Read the model definition and answer for the solid it produces. Units are mm, in the model's axes. Face numbers are marked on the shaded views. A direction names the side the tool comes from. Coordinates: 2 decimals unless noted, no trailing zeros. Order: outer loops, then holes, each group sorted by start corner. A loop starts at its lowest first (then second) coordinate and runs counter-clockwise, first axis right, second up.
```python
from build123d import *

# Parameters (mm, degrees)
SKETCH1_W           = 70.2
SKETCH1_H           = 17
SKETCH1_R           = 1.3
BOSS_EXTRUDE1_DEPTH = 1.6
SKETCH2_W           = 18.7
SKETCH2_H           = 15.5
SKETCH2_W_2         = 10.2
SKETCH2_H_2         = 14
BOSS_EXTRUDE2_DEPTH = 7.5
SKETCH3_W           = 52.2
SKETCH3_H           = 14.607054818
BOSS_EXTRUDE3_DEPTH = 2.4


with BuildPart() as part:
    # Sketch1 → Boss-Extrude1 (new body)
    with BuildSketch(Plane(origin=(0, 0, 0), x_dir=(1, 0, 0), z_dir=(0, 1, 0))):
        Rectangle(SKETCH1_W, SKETCH1_H)
        with Locations((-33.2, 6.6)):
            Circle(SKETCH1_R, mode=Mode.SUBTRACT)
        with Locations((33.2, 6.6)):
            Circle(SKETCH1_R, mode=Mode.SUBTRACT)
        with Locations((33.2, -6.6)):
            Circle(SKETCH1_R, mode=Mode.SUBTRACT)
        with Locations((-33.2, -6.6)):
            Circle(SKETCH1_R, mode=Mode.SUBTRACT)
    extrude(amount=-BOSS_EXTRUDE1_DEPTH)

    # Sketch2 → Boss-Extrude2 (add, symmetric)
    with BuildSketch(Plane.XY):
        with Locations((9.2, 7.75)):
            Rectangle(SKETCH2_W, SKETCH2_H)
        with Locations((25, 7)):
            Rectangle(SKETCH2_W_2, SKETCH2_H_2)
        with Locations((-25, 7)):
            Rectangle(SKETCH2_W_2, SKETCH2_H_2)
    extrude(amount=BOSS_EXTRUDE2_DEPTH, both=True)

    # Sketch3 → Boss-Extrude3 (add)
    with BuildSketch(Plane.XZ.offset(1.6)):
        Rectangle(SKETCH3_W, SKETCH3_H)
    extrude(amount=BOSS_EXTRUDE3_DEPTH)


solid = part.part
```
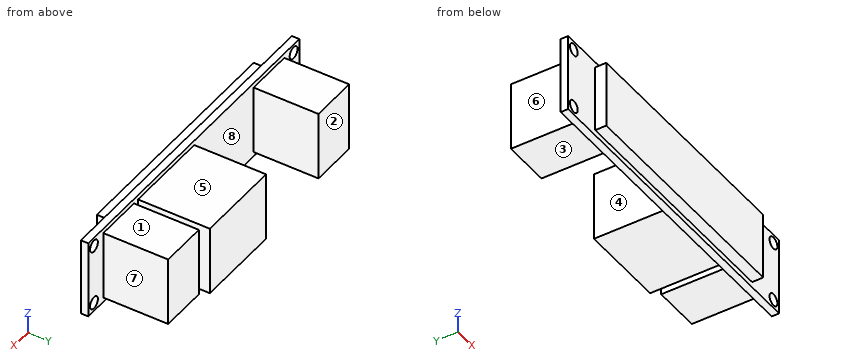
1) Flat-ended cylindrical pins translate along their axes: pin 1 Ø1.9 at (y, z) = (-2.5, 2) entering from -X; pin 2 Ø1.9 at (y, z) = (-3, -1.5) entering from +X; pin 3 Ø3 at (x, z) = (-33.2, 6.6) entering from +Y; pin 4 Ø5 at (x, z) = (-25.5, -2.5) entering from +Y. Find the tip coordinate at first contact, or state that the pin passes through.
A:
pin 1: stops at x = -35.1
pin 2: stops at x = 26.1
pin 3: stops at y = 0
pin 4: stops at y = 14
2) Which of the six approach directions +Z, -Z, +X, -X, +Y, -Y give full straight-line access (tool end or side, diameter ignored) to the marked faces 1, 2, 3 and 4?
A:
face 1: +Z, +X, -X, +Y
face 2: +Z, -Z, -X, +Y
face 3: -Z, +X, -X, +Y
face 4: +Z, -Z, +Y
3) A cutting plane is placed at B-B, the plane z = 6.6. Determine the outline of the cut face in (x, y), and give its area (3 significant figures).
A:
outline: (-35.1, -1.6) - (-34.5, -1.6) - (-34.5, 0) - (-35.1, 0) - close; (-31.9, -1.6) - (-26.1, -1.6) - (-26.1, -4) - (26.1, -4) - (26.1, -1.6) - (31.9, -1.6) - (31.9, 0) - (30.1, 0) - (30.1, 14) - (19.9, 14) - (19.9, 0) - (18.55, 0) - (18.55, 15.5) - (-0.15, 15.5) - (-0.15, 0) - (-19.9, 0) - (-19.9, 14) - (-30.1, 14) - (-30.1, 0) - (-31.9, 0) - close; (34.5, -1.6) - (35.1, -1.6) - (35.1, 0) - (34.5, 0) - close
area: 805 mm2
4) A cutting plane is placed at C-C, the plane y = 3. Determine the outline of the cut face in (x, z).
A:
outline: (-30.1, -7.5) - (-19.9, -7.5) - (-19.9, 7.5) - (-30.1, 7.5) - close; (-0.15, -7.5) - (18.55, -7.5) - (18.55, 7.5) - (-0.15, 7.5) - close; (19.9, -7.5) - (30.1, -7.5) - (30.1, 7.5) - (19.9, 7.5) - close
5) A cutting plane is placed at A-A, the plane x = -33.2. Determine the outline of the cut face in (y, z).
A:
outline: (-1.6, -8.5) - (0, -8.5) - (0, -7.9) - (-1.6, -7.9) - close; (-1.6, -5.3) - (0, -5.3) - (0, 5.3) - (-1.6, 5.3) - close; (-1.6, 7.9) - (0, 7.9) - (0, 8.5) - (-1.6, 8.5) - close
6) A cutting plane is placed at D-D, the plane y = -1. Determine the outline of the cut face in (x, z).
A:
outline: (-35.1, -8.5) - (35.1, -8.5) - (35.1, 8.5) - (-35.1, 8.5) - close; hole circle Ø2.6 at (-33.2, -6.6); hole circle Ø2.6 at (-33.2, 6.6); hole circle Ø2.6 at (33.2, -6.6); hole circle Ø2.6 at (33.2, 6.6)
7) Determine the mould class of the marked faces 5, 6, 7 and 8 for opening direction X: pulls with the +X half, pulls with the -X half, needs draft (parallel to the pull), parting line crosses it, or undercut.
A:
face 5: needs draft
face 6: pulls with the -X half
face 7: pulls with the +X half
face 8: undercut
8) Straight lines are drawn through the part: line 1 (Z direction, x = -33.2, y = -0.7); line 2 (X direction, y = 7.75, z = -4.5); line 3 (X direction, y = -0.85, z = -6.6). For each, find the intervals that lie inside material, in ascending order.
A:
line 1: z = -8.5 to -7.9, -5.3 to 5.3, 7.9 to 8.5
line 2: x = -30.1 to -19.9, -0.15 to 18.55, 19.9 to 30.1
line 3: x = -35.1 to -34.5, -31.9 to 31.9, 34.5 to 35.1
